The listing builds one solid part. Answer for the finished solid, in the listing's coordinates (mm). Face numbers are marked on the shaded views. A direction names the side the tool comes from. Give positions to 0.01 mm unless a question says otherwise; leave off trailing zeros. Order: outer loops, then holes, each group sorted by start corner. A loop starts at its lowest first (then second) coordinate and runs counter-clockwise, first axis right, second up. Notation, with made-up numbers: (-11, 10.25) - (-6, 10.25) arc R8 cw to (-6, 20.25) - close; hole circle Ø4 at (-38, -21.5). An arc over 180 degrees is marked (long way). Use CSV: the item, a comma, the result in double quotes.
```python
from build123d import *

# Parameters (mm, degrees)
BASPROSKE_W             = 7.5
BASPROSKE_H             = 4.5
TOOTHCUT_DEPTH          = 10.836157786
TEETHCUTS_COUNT         = 16
TEETHCUTS_ANGLE         = 337.5
BORSKE_R                = 2.5
BORE_DEPTH              = 50.0000508
ESQUISSE4_R             = 6
BOSS_EXTRU_3_DEPTH      = 1.9
ESQUISSE5_R             = 6.027848577
ESQUISSE5_R_2           = 2.85
BOSS_EXTRU_4_DEPTH      = 1
ESQUISSE7_R             = 3.00711341
BOSS_EXTRU_6_DEPTH      = 8.5
ESQUISSE8_R             = 7
ESQUISSE8_R_2           = 5.5
BOSS_EXTRU_7_DEPTH      = 7
BOSS_EXTRU_8_DEPTH      = 3.5
BOSS_EXTRU_8_DEPTH_BACK = 2
ESQUISSE9_R             = 13.75
ESQUISSE9_R_2           = 5.5
ESQUISSE10_R            = 1.5
ENL_V_MAT_EXTRU_3_DEPTH = 29.547066399
ESQUISSE11_R            = 3
ENL_V_MAT_EXTRU_4_DEPTH = 4
BOSS_EXTRU_9_START      = 2.1
ESQUISSE13_R            = 5.5
BOSS_EXTRU_9_DEPTH      = 10
ENL_V_START             = -4
ESQUISSE14_R            = 5.5
ENL_V_MAT_EXTRU_5_DEPTH = 4
ESQUISSE15_R            = 3.3
BOSS_EXTRU_10_DEPTH     = 14.5


with BuildPart() as part:
    # BasProSke → Base-Revolve (revolve)
    with BuildSketch(Plane(origin=(0, 0, 0), x_dir=(1, 0, 0), z_dir=(0, 1, 0)), mode=Mode.PRIVATE) as base_revolve_sk:
        with Locations((3.75, 2.25)):
            Rectangle(BASPROSKE_W, BASPROSKE_H)
    revolve(base_revolve_sk.sketch.rotate(Axis((-10, 0, 0), (1, 0, 0)), 180), axis=Axis((-10, 0, 0), (1, 0, 0)))

    # TooCutSke → ToothCut (cut, through all)
    with BuildSketch(Plane(origin=(0, 0, 0), x_dir=(0, 0, -1), z_dir=(1, 0, 0))):
        with BuildLine():
            ThreePointArc((0.306025637, 3.360092902), (0, 3.374), (-0.306025637, 3.360092902))
            ThreePointArc((-0.306025637, 3.360092902), (-0.415941512, 3.953968919), (-0.738171669, 4.464789776))
            ThreePointArc((-0.738171669, 4.464789776), (0, 4.5254), (0.738171669, 4.464789776))
            ThreePointArc((0.738171669, 4.464789776), (0.415941512, 3.953968919), (0.306025637, 3.360092902))
        make_face()
    toothcut = extrude(amount=TOOTHCUT_DEPTH, mode=Mode.SUBTRACT)

    # TeethCuts: ToothCut ×16 about axis
    teethcuts_axis = Axis((-10, 0, 0), (1, 0, 0))
    for i in range(1, TEETHCUTS_COUNT):
        add(toothcut.rotate(teethcuts_axis, i * TEETHCUTS_ANGLE / (TEETHCUTS_COUNT - 1)), mode=Mode.SUBTRACT)

    # BorSke → Bore (cut, symmetric)
    with BuildSketch(Plane(origin=(0, 0, 0), x_dir=(0, 0, -1), z_dir=(1, 0, 0))):
        with Locations(Location((0, 0, 0), (0, 0, 180))):
            Circle(BORSKE_R)
    extrude(amount=BORE_DEPTH, both=True, mode=Mode.SUBTRACT)

    # Esquisse4 → Boss.-Extru.3 (add)
    with BuildSketch(Plane.ZY):
        with Locations(Location((0, 0, 0), (0, 0, 180))):
            Circle(ESQUISSE4_R)
    extrude(amount=BOSS_EXTRU_3_DEPTH)

    # Esquisse5 → Boss.-Extru.4 (add)
    with BuildSketch(Plane(origin=(7.5, 0, 0), x_dir=(0, 0, -1), z_dir=(1, 0, 0))):
        Circle(ESQUISSE5_R)
        Circle(ESQUISSE5_R_2, mode=Mode.SUBTRACT)
    extrude(amount=BOSS_EXTRU_4_DEPTH)

    # Esquisse7 → Boss.-Extru.6 (add)
    with BuildSketch(Plane(origin=(0, 0, 0), x_dir=(0, 0, -1), z_dir=(1, 0, 0))):
        Circle(ESQUISSE7_R)
    extrude(amount=BOSS_EXTRU_6_DEPTH)

    # Esquisse8 → Boss.-Extru.7 (add)
    with BuildSketch(Plane.ZY.offset(1.9)):
        Circle(ESQUISSE8_R)
        Circle(ESQUISSE8_R_2, mode=Mode.SUBTRACT)
    extrude(amount=BOSS_EXTRU_7_DEPTH)

    # Esquisse9 → Boss.-Extru.8 (add, two sides: drawn at the far end of the back side and taken through both)
    with BuildSketch(Plane.ZY.offset(8.9).offset(-BOSS_EXTRU_8_DEPTH_BACK)):
        Circle(ESQUISSE9_R)
        Circle(ESQUISSE9_R_2, mode=Mode.SUBTRACT)
    extrude(amount=BOSS_EXTRU_8_DEPTH + BOSS_EXTRU_8_DEPTH_BACK)

    # Esquisse10 → Enlèv. mat.-Extru.3 (cut, through all)
    with BuildSketch(Plane.ZY.offset(12.4)):
        with Locations((0, 11.3)):
            Circle(ESQUISSE10_R)
        with Locations((0, -11.3)):
            Circle(ESQUISSE10_R)
    extrude(amount=-ENL_V_MAT_EXTRU_3_DEPTH, mode=Mode.SUBTRACT)

    # Esquisse11 → Enlèv. mat.-Extru.4 (cut)
    with BuildSketch(Plane.ZY.offset(1.9)):
        Circle(ESQUISSE11_R)
    extrude(amount=-ENL_V_MAT_EXTRU_4_DEPTH, mode=Mode.SUBTRACT)

    # Esquisse13 → Boss.-Extru.9 (add)
    with BuildSketch(Plane.ZY.offset(-2.1).offset(BOSS_EXTRU_9_START)):
        Circle(ESQUISSE13_R)
    extrude(amount=BOSS_EXTRU_9_DEPTH)

    # Esquisse14 → Enlèv. mat.-Extru.5 (cut)
    with BuildSketch(Plane.ZY.offset(10).offset(ENL_V_START)):
        Circle(ESQUISSE14_R)
    extrude(amount=ENL_V_MAT_EXTRU_5_DEPTH, mode=Mode.SUBTRACT)

    # Esquisse15 → Boss.-Extru.10 (add)
    with BuildSketch(Plane.ZY.offset(6)):
        Circle(ESQUISSE15_R)
    extrude(amount=-BOSS_EXTRU_10_DEPTH)


solid = part.part
```
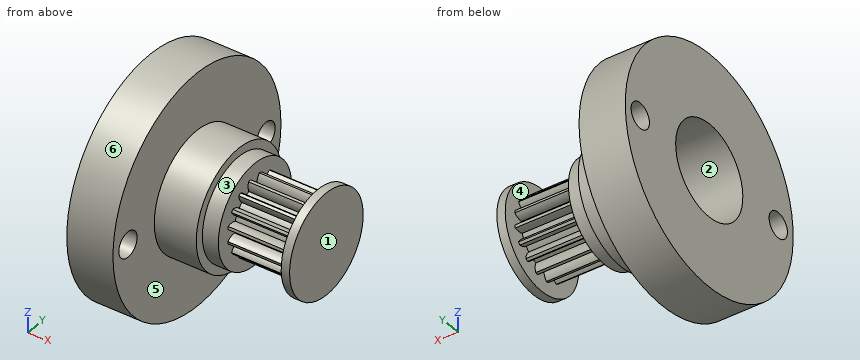
Item 1: The mould has two halves that part along Z. Classify the marked faces 1, 2 and 3: +Z half, -Z half, draft (parallel to the pull), parting line (faces both ways), or undercut.
Taken from the geometry:
face 1,"draft"
face 2,"undercut"
face 3,"parting line"
Item 2: Which of the six approach directions +Z, -Z, +X, -X, +Y, -Y give full straight-line access (tool end or side, diameter ignored) to the marked faces 4, 5 and 6?
Taken from the geometry:
face 4,"none"
face 5,"+X"
face 6,"+X, -X"
Item 3: The part is cut by section B-B (x = -6.5). Give the vertices of the cut face in (y, z).
Taken from the geometry:
outline,"circle Ø14 at (0, 0); hole circle Ø11 at (0, 0)"
Item 4: The part is cut by section C-C (z = -6.5). Give the vertices of the cut face in (x, y), and give its area (3 significant figures).
Taken from the geometry:
outline,"(-12.4, -12.12) - (-6.9, -12.12) - (-6.9, -2.6) - (-1.9, -2.6) - (-1.9, 2.6) - (-6.9, 2.6) - (-6.9, 12.12) - (-12.4, 12.12) - close"
area,"159 mm^2"
Item 5: Find the intervals of material crossed by line 1 along Y through (x, z) = (-10.75, 0); line 2 along X through (y, z) = (-4.5, 10.5); line 3 along Y through (x, z) = (-5.75, 3.75), in increasing order.
Taken from the geometry:
line 1,"-13.75 to -12.8, -9.8 to -5.5, 5.5 to 9.8, 12.8 to 13.75"
line 2,"-12.4 to -6.9"
line 3,"-5.91 to 5.91"
Item 6: Each of these flat-tipped pins is pushed along its axis until it touches: pin 1 (12 mm diameter, centred on x = 3, z = 1, fed in from -Y); pin 2 (6 mm diameter, centred on x = -3, z = -9, fed in from -Y); pin 3 (12 mm diameter, centred on x = 2.5, y = 8.5, fed in from +Z). Where does it stop, or does it pass through?
Taken from the geometry:
pin 1,"y = -7"
pin 2,"y = -3.61"
pin 3,"z = 5.43"
Item 7: The part is cut by section A-A (y = -11.3). Give the vertices of the cut face in (x, z).
Taken from the geometry:
outline,"(-12.4, -7.83) - (-6.9, -7.83) - (-6.9, -1.5) - (-12.4, -1.5) - close; (-12.4, 1.5) - (-6.9, 1.5) - (-6.9, 7.83) - (-12.4, 7.83) - close"
Item 8: The part is cut by section D-D (x = -1). Give the vertices of the cut face in (y, z).
Taken from the geometry:
outline,"circle Ø12 at (0, 0)"
